Geometry: final body of the model. Coordinates: model frame, mm. Face numbers are marked on the shaded views. A direction names the side the tool comes from. Give positions to 0.01 mm unless a question says otherwise; leave off trailing zeros. Write each loop counter-clockwise with the first axis right and the second up, starting at its lowest first coordinate (ties: lowest second). Pieces come first, ordered by that corner, then holes. Notation, with made-up numbers: (13, 53.25) - (51, 53.25) arc R33 cw to (51, 81.25) - close; hole circle Ø2 at (74.25, 3). An arc over 180 degrees is marked (long way). Use CSV: the item, a comma, the result in double quotes. Start each with the question number.
(1) Section D-D on x = 25. Output: boundary loops of the cut face in (y, z).
(2) Section C-C on z = 23. Output: boundary loops of the cut face in (x, y).
(3) First-contact query: pin 1 Ø5 at (x, z) = (41.33, 0) entering from +Y; pin 2 Ø10 at (x, y) = (23.5, -20) entering from -Z; pin 3 Ø5 at (x, z) = (12, -1) entering from +Y; pin 4 Ø6 at (y, z) = (-4, 33.5) entering from +X. Flat tips, straight axial feed; report the tip coordinate or a pass-through.
(4) Reachability of the marked faces 4, 5 and 6 from +Z, -Z, +X, -X, +Y, -Y: full face, straight path, thin tool, end or side. Return the list, or none.
(5) Line query: probe 1 along Z at (x, y) = (33.5, -20.5); probe 2 along X at (y, z) = (-9.5, 43); probe 3 along Z at (x, y) = (-23.5, -3.75). Output: solid intervals per line, ascending. Write a range as [from, to].
(6) Section B-B on x = 41. Output: boundary loops of the cut face in (y, z).
(7) Draft query along X for the marked faces 1, 2 and 3. Return one class per face: released by +X, released by -X, zero draft, split by the parting line, or undercut.
(8) Section A-A on z = 0. Output: boundary loops of the cut face in (x, y).
from build123d import *

# Parameters (mm, degrees)
F0_W     = 74.4671411812
F0_H     = 53.2596688718
F1_DEPTH = 25.4
F3_DEPTH = 74.676
F4_DEPTH = 96.012
F5_DEPTH = 126.238
F6_R     = 2.8919279575
F7_DEPTH = 69.596
F8_R     = 2.7844971125
F9_DEPTH = 71.374


with BuildPart() as f1:
    # F0 (on Front) → F1 (new body)
    with BuildSketch(Plane.XZ):
        with Locations((9.880753234, 0.4819883034)):
            Rectangle(F0_W, F0_H)
    extrude(amount=F1_DEPTH)

    # F2 (on face) → F3 (join)
    with BuildSketch(Plane.XY.offset(27.1118227392)):
        with BuildLine():
            ThreePointArc((36.5105904639, 0), (11.0857244581, -12.4089535166), (-14.3391415477, 0))
            Line((-14.3391415477, 0), (-20.1229974627, 0))
            ThreePointArc((-20.1229974627, 0), (10.9652262181, -16.6939246271), (42.053449899, 0))
            Line((42.053449899, 0), (36.5105904639, 0))
        make_face()
    extrude(amount=-F3_DEPTH)

    # F4 (add): a face of the model
    f4_faces = [f1.faces().sort_by_distance(p)[0] for p in [
        (39.2820201814, -0.643785502, -47.5641772608),
    ]]
    extrude(f4_faces, amount=-F4_DEPTH)

    # F5 (cut): a face of the model
    f5_faces = [f1.faces().sort_by_distance(p)[0] for p in [
        (11.0857244581, -5.0557746848, 27.1118227392),
    ]]
    extrude(f5_faces, amount=-F5_DEPTH, mode=Mode.SUBTRACT)

    # F6 (on face) → F7 (cut)
    with BuildSketch(Plane(origin=(0, 0, 0), x_dir=(-1, 0, 0), z_dir=(0, 1, 0))):
        with Locations((23.0149254203, 0)):
            Circle(F6_R)
    extrude(amount=-F7_DEPTH, mode=Mode.SUBTRACT)

    # F8 (on face) → F9 (cut)
    with BuildSketch(Plane(origin=(0, 0, 0), x_dir=(-1, 0, 0), z_dir=(0, 1, 0))):
        with Locations((-41.3304679096, 0)):
            Circle(F8_R)
    extrude(amount=-F9_DEPTH, mode=Mode.SUBTRACT)


solid = f1.part
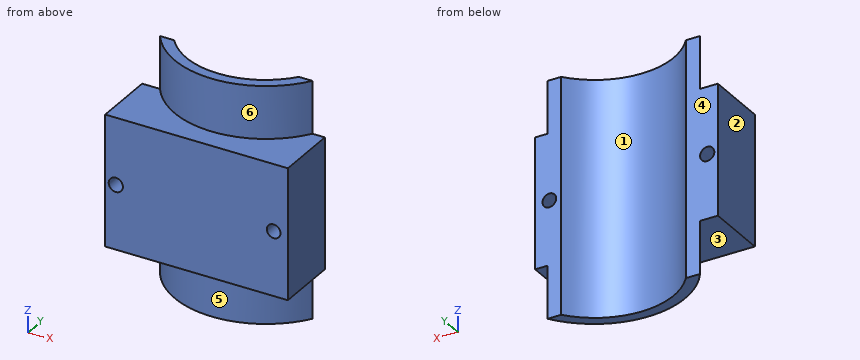
Check values:
1,outline,"(-25.4, -26.15) - (-13.95, -26.15) - (-13.95, -47.56) - (-9.25, -47.56) - (-9.25, 48.45) - (-13.95, 48.45) - (-13.95, 27.11) - (-25.4, 27.11) - close"
2,outline,"(-27.35, -25.4) - (47.11, -25.4) - (47.11, 0) - (36.51, 0) arc R32.25 cw to (-14.34, 0) - (-27.35, 0) - close"
3,pin 1,"passes through"
3,pin 2,"stops at z = -26.15"
3,pin 3,"stops at y = -12.23"
3,pin 4,"stops at x = 41.37"
4,face 4,"+Z, -Z, +X, -X, +Y"
4,face 5,"-Z, -Y"
4,face 6,"+Z, -Y"
5,probe 1,"z = [-26.15, 27.11]"
5,probe 2,"x = [-11.05, -2.3], [24.47, 32.98]"
5,probe 3,"z = [-26.15, -2.85], [2.85, 27.11]"
6,outline,"(-25.4, -26.15) - (-1.51, -26.15) - (-1.51, -47.56) - (0, -47.56) - (0, -2.76) - (-25.4, -2.76) - close; (-25.4, 2.76) - (0, 2.76) - (0, 48.45) - (-1.51, 48.45) - (-1.51, 27.11) - (-25.4, 27.11) - close"
7,face 1,"undercut"
7,face 2,"released by -X"
7,face 3,"zero draft"
8,outline,"(-27.35, -25.4) - (-25.91, -25.4) - (-25.91, 0) - (-27.35, 0) - close; (-20.12, -25.4) - (38.55, -25.4) - (38.55, 0) - (36.51, 0) arc R32.25 cw to (-14.34, 0) - (-20.12, 0) - close; (44.11, -25.4) - (47.11, -25.4) - (47.11, 0) - (44.11, 0) - close"
